Source: CAD feature listing. Evaluate the final solid. Frame: model axes, mm. A direction names the side the tool comes from. Round coordinates to 2 decimals unless told otherwise and drop trailing zeros. Order: outer loops, then holes, each group sorted by start corner. A loop starts at its lowest first (then second) coordinate and runs counter-clockwise, first axis right, second up. Notation, with made-up numbers: (61, -6.5) - (66, -6.5) arc R13 cw to (66, -2.5) - close; hole circle Ø11 at (-28.5, 20.5). An arc over 180 degrees is marked (long way). Use one line per item in the form item = value. Start each with the question number.
Q1. Set-up query: faces 4 (the cylindrical face through (-0.553, -39.214, 109.831)), 5 (the cylindrical face through (-35.17, -39.6, 259.43)), 6 (the cylindrical face through (-4.506, 64.822, 131.693)), 7 (the flat face through (83, 0, 84)), 8 (the flat face through (59, 17, 158)). Return all of +Z, -Z, +X, -X, +Y, -Y with unobstructed straight access to the full face (end or side cutting, diameter ignored); none if empty.
Q2. Pin query (flat end, axial travel): pin 1 Ø16 at (x, y) = (66.47, -66.47) entering from +Z; pin 2 Ø1 at (x, y) = (-67.5, -46.5) entering from -Z; pin 3 Ø5 at (x, z) = (77.5, 55) entering from +Y; pin 4 Ø12.5 at (x, z) = (0, 252) entering from -Y. Return the tip coordinate at first contact, or that it passes through.
Q3. Cut plane A-A, the plane z = 57.5. Return the cut outline in (x, y).
Q4. Ray query, line 1 (Z direction, x = -33, y = 24); line 2 (Z direction, x = -7.5, y = -31); line 3 (Z direction, x = 5, y = -53.5). Return the intervals inside material, ascending. Write a range as [from, to].
Q5. Draft query along X for faces 1 (the cylindrical face through (-62.44, -2.75, -1.48)), 2 (the flat face through (4, 76, 247)), 3 (the cylindrical face through (56, 0, 70)). Return one class per face: released by +X, released by -X, zero draft, split by the parting line, or undercut.
Q6. Cut plane B-B, the plane x = 99. Return the cut outline in (y, z), and give its area (3 significant figures).
from build123d import *

# Parameters (mm, degrees)
SKETCH_1_R               = 114
EXTRUDE_1_DEPTH          = 12
EXTRUDE_START            = 258
SKETCH_2_R               = 62.5
EXTRUDE_2_DEPTH          = 28
SKETCH_3_R               = 56
EXTRUDE_3_DEPTH          = 112
SKETCH_4_R               = 30
EXTRUDE_4_DEPTH          = 28
EXTRUDE_5_REACH          = 234.843
EXTRUDE_6_DEPTH          = 118
EXTRUDE_18_DEPTH         = 28
EXTRUDE_19_DEPTH         = 10
SKETCH_12_R              = 15
EXTRUDE_20_DEPTH         = 76
SKETCH_13_R              = 15
EXTRUDE_21_DEPTH         = 76
SKETCH_14_R              = 9
CUT_EXTRUDE_1_DEPTH      = 305.230176103
PATTERN_CIRCULAR_1_COUNT = 4
SKETCH_15_R              = 62.5
EXTRUDE_22_DEPTH         = 3
SKETCH_16_R              = 37.5
CUT_EXTRUDE_2_DEPTH      = 128
PATTERN_CIRCULAR_2_COUNT = 4
SKETCH_19_R              = 41
CUT_EXTRUDE_3_DEPTH      = 8
SKETCH_20_R              = 15
EXTRUDE_23_DEPTH         = 3
CUT_EXTRUDE_4_REACH      = 220.852
SKETCH_21_R              = 12
SKETCH_22_R              = 18
CUT_EXTRUDE_5_DEPTH      = 28
CHAMFER_1_SIZE           = 6.92820323
CHAMFER_1_SIZE_2         = 4
F_1_4_RC_1_AT_2_COUNT    = 2
F_1_4_RC_1_AT_2_PITCH    = 106
F_5_0MM_START            = 11.779218889
F_5_0MM_1_OUTLINE_R      = 2.5
F_5_0MM_1_DEPTH          = 47.722932759
SKETCH_26_R              = 15
SKETCH_26_R_2            = 12
EXTRUDE_24_DEPTH         = 3


# Read off the part's stored shape, not the designer's step: the hole wizard step, the hole wizard step
with BuildPart() as part:
    # Sketch 1 → Extrude 1 (new body)
    with BuildSketch(Plane.XY):
        Circle(SKETCH_1_R)
    extrude(amount=EXTRUDE_1_DEPTH)

    # Sketch 6 → Extrude 6 (add)
    with BuildSketch(Plane.XY.offset(12)):
        with BuildLine():
            Line((51.396417147, 22.235294118), (62.409935107, 27))
            ThreePointArc((62.409935107, 27), (65.390118151, 18.658307753), (67.260686883, 10))
            Line((67.260686883, 10), (83, 10))
            Line((83, 10), (83, -10))
            Line((83, -10), (67.260686883, -10))
            ThreePointArc((67.260686883, -10), (65.390118151, -18.658307753), (62.409935107, -27))
            Line((62.409935107, -27), (51.396417147, -22.235294118))
            ThreePointArc((51.396417147, -22.235294118), (56, 0), (51.396417147, 22.235294118))
        make_face()
    extrude_6 = extrude(amount=EXTRUDE_6_DEPTH)



with BuildPart() as body_2:
    # Sketch 2 → Extrude 2 (new body)
    with BuildSketch(Plane.XY.offset(12).offset(EXTRUDE_START)):
        Circle(SKETCH_2_R)
    extrude(amount=-EXTRUDE_2_DEPTH)

    # Sketch 3 → Extrude 3 (add)
    with BuildSketch(Plane(origin=(0, 0, 242), x_dir=(-1, 0, 0), z_dir=(0, 0, -1))):
        Circle(SKETCH_3_R)
    extrude(amount=EXTRUDE_3_DEPTH)

    # Sketch 4 → Extrude 4 (add)
    with BuildSketch(Plane(origin=(0, 0, 130), x_dir=(-1, 0, 0), z_dir=(0, 0, -1))):
        Circle(SKETCH_4_R)
    extrude(amount=EXTRUDE_4_DEPTH)

    # Sketch 5 → Extrude 5 (add, up to next)
    with BuildSketch(Plane(origin=(0, 0, 102), x_dir=(-1, 0, 0), z_dir=(0, 0, -1)), mode=Mode.PRIVATE) as extrude_5_sk1:
        with BuildLine():
            ThreePointArc((-26.681798428, 13.714285714), (0, 30), (26.681798428, 13.714285714))
            Line((26.681798428, 13.714285714), (12.451505933, 41.4))
            ThreePointArc((12.451505933, 41.4), (0, 49), (-12.451505933, 41.4))
            Line((-12.451505933, 41.4), (-26.681798428, 13.714285714))
        make_face()
    extrude_5_tool1 = extrude(extrude_5_sk1.sketch, amount=-EXTRUDE_5_REACH, mode=Mode.PRIVATE) - body_2.part
    # Sketch 5 → Extrude 5 (add, up to next)
    with BuildSketch(Plane(origin=(0, 0, 102), x_dir=(-1, 0, 0), z_dir=(0, 0, -1)), mode=Mode.PRIVATE) as extrude_5_sk2:
        with BuildLine():
            Line((12.451505933, -41.4), (26.681798428, -13.714285714))
            ThreePointArc((26.681798428, -13.714285714), (0, -30), (-26.681798428, -13.714285714))
            Line((-26.681798428, -13.714285714), (-12.451505933, -41.4))
            ThreePointArc((-12.451505933, -41.4), (0, -49), (12.451505933, -41.4))
        make_face()
    extrude_5_tool2 = extrude(extrude_5_sk2.sketch, amount=-EXTRUDE_5_REACH, mode=Mode.PRIVATE) - body_2.part
    add(extrude_5_tool1.solids().sort_by_distance((0, 35.767419, 102))[0])
    add(extrude_5_tool2.solids().sort_by_distance((0, -35.767419, 102))[0])


with BuildPart() as part_1:
    add(part.part)

    add(body_2.part)  # Extrude 18 merges body 2
    # Sketch 10 → Extrude 18 (add)
    with BuildSketch(Plane.XY.offset(130)):
        with BuildLine():
            Line((51.396417147, -22.235294118), (62.409935107, -27))
            ThreePointArc((62.409935107, -27), (65.390118151, -18.658307753), (67.260686883, -10))
            Line((67.260686883, -10), (83, -10))
            Line((83, -10), (83, 10))
            Line((83, 10), (67.260686883, 10))
            ThreePointArc((67.260686883, 10), (65.390118151, 18.658307753), (62.409935107, 27))
            Line((62.409935107, 27), (51.396417147, 22.235294118))
            ThreePointArc((51.396417147, 22.235294118), (56, 0), (51.396417147, -22.235294118))
        make_face()
    extrude_18 = extrude(amount=EXTRUDE_18_DEPTH)

    # Sketch 11 → Extrude 19 (add, symmetric)
    with BuildSketch(Plane(origin=(0, 0, 0), x_dir=(1, 0, 0), z_dir=(0, 1, 0))):
        with BuildLine():
            Line((51.396417147, -189.603582853), (51.396417147, -158))
            Line((51.396417147, -158), (83, -158))
            ThreePointArc((83, -158), (73.743524892, -180.347107745), (51.396417147, -189.603582853))
        make_face()
    extrude_19 = extrude(amount=EXTRUDE_19_DEPTH, both=True)

    # Mirror 4: Extrude 6, Extrude 18, Extrude 19 across plane
    add(extrude_6.mirror(Plane(origin=(0, 0, 0), x_dir=(0, 0, 1), z_dir=(1, 0, 0))))
    add(extrude_18.mirror(Plane(origin=(0, 0, 0), x_dir=(0, 0, 1), z_dir=(1, 0, 0))))
    add(extrude_19.mirror(Plane(origin=(0, 0, 0), x_dir=(0, 0, 1), z_dir=(1, 0, 0))))

    # Sketch 12 → Extrude 20 (add)
    with BuildSketch(Plane(origin=(0, 0, 0), x_dir=(1, 0, 0), z_dir=(0, 1, 0))):
        with Locations(Location((0, -252, 0), (0, 0, 138.189685104))):
            Circle(SKETCH_12_R)
    extrude(amount=EXTRUDE_20_DEPTH)

    # Sketch 13 → Extrude 21 (add)
    with BuildSketch(Plane(origin=(0, 0, 0), x_dir=(1, 0, 0), z_dir=(0, 1, 0))):
        with Locations(Location((0, -146, 0), (0, 0, 90))):
            Circle(SKETCH_13_R)
    extrude(amount=EXTRUDE_21_DEPTH)

    # Sketch 14 → Cut-Extrude 1 (cut, through all)
    with BuildSketch(Plane.XY.offset(12)):
        with Locations((66.468037432, -66.468037432)):
            Circle(SKETCH_14_R)
    cut_extrude_1 = extrude(amount=-CUT_EXTRUDE_1_DEPTH, mode=Mode.SUBTRACT)

    # Pattern Circular 1: Cut-Extrude 1 ×4 about axis
    pattern_circular_1_axis = Axis((-0.436506366, 0.436506366, 0), (0, 0, 1))
    for i in range(1, PATTERN_CIRCULAR_1_COUNT):
        add(cut_extrude_1.rotate(pattern_circular_1_axis, i * 360 / PATTERN_CIRCULAR_1_COUNT), mode=Mode.SUBTRACT)

    # Sketch 15 → Extrude 22 (add)
    with BuildSketch(Plane(origin=(0, 0, 0), x_dir=(-1, 0, 0), z_dir=(0, 0, -1))):
        with Locations(Location((0, 0, 0), (0, 0, 180))):
            Circle(SKETCH_15_R)
    extrude(amount=EXTRUDE_22_DEPTH)

    # Sketch 16 → Cut-Extrude 2 (cut)
    with BuildSketch(Plane.XY.offset(270)):
        Circle(SKETCH_16_R)
    extrude(amount=-CUT_EXTRUDE_2_DEPTH, mode=Mode.SUBTRACT)

    # Sketch 18 → Hole Wizard M10 _1 (revolve, cut)
    with BuildSketch(Plane(origin=(35.355339059, 35.355339059, 270), x_dir=(0, -1, 0), z_dir=(1, 0, 0))):
        Polygon((0, 0), (0, 24), (4.25, 21.446342369), (4.25, 0), align=None)
    hole_wizard_m10_1 = revolve(axis=Axis((35.355339059, 35.355339059, 276.35), (0, 0, -1)), mode=Mode.SUBTRACT)

    # Pattern Circular 2: Hole Wizard M10 _1 ×4 about axis
    pattern_circular_2_axis = Axis((0, 0, 0), (0, 0, 1))
    for i in range(1, PATTERN_CIRCULAR_2_COUNT):
        add(hole_wizard_m10_1.rotate(pattern_circular_2_axis, i * 360 / PATTERN_CIRCULAR_2_COUNT), mode=Mode.SUBTRACT)

    # Sketch 19 → Cut-Extrude 3 (cut)
    with BuildSketch(Plane.XY.offset(142)):
        Circle(SKETCH_19_R)
    extrude(amount=CUT_EXTRUDE_3_DEPTH, mode=Mode.SUBTRACT)

    # Sketch 20 → Extrude 23 (add)
    with BuildSketch(Plane.XY.offset(142)):
        Circle(SKETCH_20_R)
    extrude(amount=EXTRUDE_23_DEPTH)

    # Sketch 21 → Cut-Extrude 4 (cut, up to next)
    with BuildSketch(Plane.XY.offset(145), mode=Mode.PRIVATE) as cut_extrude_4_sk1:
        Circle(SKETCH_21_R)
    cut_extrude_4_tool1 = extrude(cut_extrude_4_sk1.sketch, amount=-CUT_EXTRUDE_4_REACH, mode=Mode.PRIVATE) & part_1.part
    add(cut_extrude_4_tool1.solids().sort_by_distance((0, 0, 145))[0], mode=Mode.SUBTRACT)

    # Sketch 22 → Cut-Extrude 5 (cut)
    with BuildSketch(Plane(origin=(0, 0, 102), x_dir=(-1, 0, 0), z_dir=(0, 0, -1))):
        Circle(SKETCH_22_R)
    extrude(amount=-CUT_EXTRUDE_5_DEPTH, mode=Mode.SUBTRACT)

    # Chamfer 1
    # the kernel refuses this chamfer: 6.92820323, 4 mm, written as the material it takes off along each edge
    with BuildSketch(Plane(origin=(0, 0, 130), x_dir=(1, 0, 0), z_dir=(0, -1, 0))) as chamfer_1_piece_1_section:
        Polygon((12 + CHAMFER_1_SIZE, 0), (12, CHAMFER_1_SIZE_2), (12, 0), align=None)
    chamfer_1_piece_1 = revolve(axis=Axis((0, 0, 130), (0, 0, 1)), mode=Mode.PRIVATE)
    chamfer_1_piece_1 = chamfer_1_piece_1 & Plane(origin=(0, 0, 132.241387072), x_dir=(-1, 0, 0), z_dir=(0, 0, -1)) * Cylinder(18, 76, mode=Mode.PRIVATE)
    add(chamfer_1_piece_1, mode=Mode.SUBTRACT)

    # Sketch 24 → 1_4 Rc _1 (revolve, cut)
    with BuildSketch(Plane(origin=(0, 76, 252), x_dir=(0, 0, 1), z_dir=(1, 0, 0))):
        Polygon((0, 0), (0, 18), (5.35, 14.785395688), (5.35, 14), (5.810617305, 14), (6.24765, 0), align=None)
    f_1_4_rc_1 = revolve(axis=Axis((0, 82.35, 252), (0, -1, 0)), mode=Mode.SUBTRACT)

    # 1_4 Rc _1 at 2: 1_4 Rc _1 ×2
    with Locations(*[(0, 0, -i * F_1_4_RC_1_AT_2_PITCH) for i in range(1, F_1_4_RC_1_AT_2_COUNT)]):
        add(f_1_4_rc_1, mode=Mode.SUBTRACT)

    # 5.0mm _1 outline → 5.0mm _1 (cut)
    with BuildSketch(Plane(origin=(0, 0, 0), x_dir=(1, 0, 0), z_dir=(0, 1, 0)).offset(F_5_0MM_START)):
        with Locations((0, -252)):
            Circle(F_5_0MM_1_OUTLINE_R)
        with BuildLine():
            ThreePointArc((-2.291287847, -145), (0, -148.5), (2.291287847, -145))
            ThreePointArc((2.291287847, -145), (0, -143.5), (-2.291287847, -145))
        make_face()
    extrude(amount=F_5_0MM_1_DEPTH, mode=Mode.SUBTRACT)

    # Sketch 26 → Extrude 24 (add)
    with BuildSketch(Plane.XY.offset(145)):
        Circle(SKETCH_26_R)
        Circle(SKETCH_26_R_2, mode=Mode.SUBTRACT)
    extrude(amount=-EXTRUDE_24_DEPTH)

    # Hole Wizard M10 _2 outline → Hole Wizard M10 _2 (revolve, cut)
    with BuildSketch(Plane.XZ.offset(-35)):
        Polygon((4.25, 117.446342369), (0, 120), (0, 102), (4.25, 102), align=None)
    hole_wizard_m10_2 = revolve(axis=Axis((0, 35, 0), (0, 0, 1)), mode=Mode.SUBTRACT)

    # Mirror 6: Hole Wizard M10 _2 across plane
    add(hole_wizard_m10_2.mirror(Plane.ZX), mode=Mode.SUBTRACT)


solid = part_1.part
Completed:
q1.face_4 = none
q1.face_5 = +Z
q1.face_6 = +Y
q1.face_7 = +Z, +X, +Y, -Y
q1.face_8 = +X, +Y
q2.pin_1 = through
q2.pin_2 = 0
q2.pin_3 = 10
q2.pin_4 = -62.5
q3.outline = (-83, -10) - (-67.26, -10) arc R68 ccw to (-62.41, -27) - (-51.4, -22.24) arc R56 cw to (-51.4, 22.24) - (-62.41, 27) arc R68 ccw to (-67.26, 10) - (-83, 10) - close; (51.4, -22.24) - (62.41, -27) arc R68 ccw to (67.26, -10) - (83, -10) - (83, 10) - (67.26, 10) arc R68 ccw to (62.41, 27) - (51.4, 22.24) arc R56 cw to start
q4.line_1 = [-3, 12], [130, 142], [150, 270]
q4.line_2 = [-3, 12], [102, 142]
q4.line_3 = [-3, 12], [130, 270]
q5.face_1 = split by the parting line
q5.face_2 = zero draft
q5.face_3 = undercut
q6.outline = (-56.52, 0) - (56.52, 0) - (56.52, 12) - (-56.52, 12) - close
q6.area = 1,360 mm2
